Part print with two shaded views. Sizes in mm from the minimum x, y, z corner. Coordinates: 2 decimals unless noted, no trailing zeros. Order: outer loops, then holes, each group sorted by start corner. A loop starts at its lowest first (then second) coordinate and runs counter-clockwise, first axis right, second up. Notation, with made-up numbers: (81.5, 37) - (105.5, 37) arc R26 ccw to (105.5, 65) - close; hole circle Ø6 at (-32.75, 20). An arc over 180 degrees is marked (long way). One line per item, written item: value.
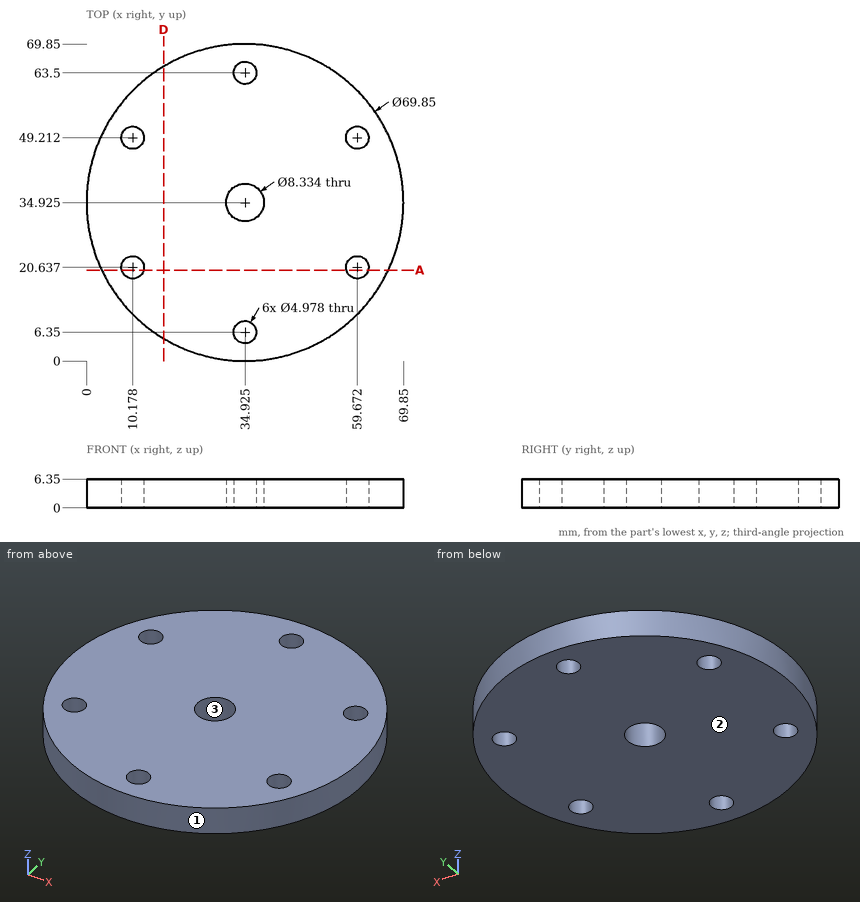
1. Probe line 1 along Y through (x, z) = (10.5, 2.25) (1 decimal); line 2 along Y through (x, z) = (33.5, 1); line 3 along Y through (x, z) = (59, 4.5) (1 decimal). List the from-to ranges inside material, lowest first.
Values found:
line 1: y = 10 to 18.2, 23.1 to 46.7, 51.7 to 59.9
line 2: y = 0.03 to 4.31, 8.39 to 31.01, 38.84 to 61.46, 65.54 to 69.82
line 3: y = 9.6 to 18.2, 23 to 46.8, 51.6 to 60.2
2. Flat gauge pins, fed straight in: P1, Ø4, axis at x = 8.5, y = 12.5, coming from the -Z side; P2, Ø2, axis at y = 18, z = 2, coming from the -X side; P3, Ø3, axis at x = 14.5, z = 2.5, coming from the +Y side; P4, Ø1, axis at x = 52.5, z = 2, coming from the -Y side. Where does each tip first touch, or does it go through?
Values found:
P1: stops at z = 0
P2: stops at x = 3.84
P3: stops at y = 64.28
P4: stops at y = 4.46
3. Band-saw the part on D-D, the plane x = 17. Give the cut face in (y, z).
Values found:
outline: (4.95, 0) - (64.9, 0) - (64.9, 6.35) - (4.95, 6.35) - close
4. Two-plate mould, pull along X, no slides. Class the marked faces 1, 2 and 3: pulls with the +X half, pulls with the -X half, needs draft (parallel to the pull), parting line crosses it, or undercut.
Values found:
face 1: parting line crosses it
face 2: needs draft
face 3: undercut
5. Band-saw the part on A-A, the plane y = 20. Count the separate pieces of the cut face and the enclosed holes in it, and give its area (3 significant figures).
Values found:
separate pieces: 3
enclosed holes: 0
area: 340 mm2
